Geometry check sheet. Reference: the model listing, model coordinates, mm. A direction names the side the tool comes from. Round coordinates to 2 decimals unless told otherwise and drop trailing zeros. Answer in a Markdown table with one row per item. Add a question column.
from build123d import *

# Parameters (mm, degrees)
SKETCH1_W                                           = 300
SKETCH1_H                                           = 180
BOSS_EXTRUDE1_DEPTH                                 = 10
CBORE_FOR_4_BINDING_HEAD_MACHINE_SCREW1_D           = 3.2639
CBORE_FOR_4_BINDING_HEAD_MACHINE_SCREW1_DEPTH       = 10
CBORE_FOR_4_BINDING_HEAD_MACHINE_SCREW1_CBORE_D     = 6.74624
CBORE_FOR_4_BINDING_HEAD_MACHINE_SCREW1_CBORE_DEPTH = 1.7272


with BuildPart() as part:
    # Sketch1 → Boss-Extrude1 (new body)
    with BuildSketch(Plane(origin=(0, 0, 0), x_dir=(1, 0, 0), z_dir=(0, 1, 0))):
        with Locations((21.639344262, -12.295081967)):
            Rectangle(SKETCH1_W, SKETCH1_H)
    extrude(amount=BOSS_EXTRUDE1_DEPTH)

    # CBORE for #4 Binding Head Machine Screw1
    with Locations(Plane(origin=(0, 10, 0), x_dir=(1, 0, 0), z_dir=(0, 1, 0))):
        with Locations((-123.360655738, 37.704918033), (-123.360655738, -62.295081967), (-78.360655738, -97.295081967), (121.639344262, -97.295081967), (121.639344262, 72.704918033), (166.639344262, 37.704918033), (-78.360655738, 72.704918033)):
            CounterBoreHole(CBORE_FOR_4_BINDING_HEAD_MACHINE_SCREW1_D / 2, CBORE_FOR_4_BINDING_HEAD_MACHINE_SCREW1_CBORE_D / 2, CBORE_FOR_4_BINDING_HEAD_MACHINE_SCREW1_CBORE_DEPTH, depth=CBORE_FOR_4_BINDING_HEAD_MACHINE_SCREW1_DEPTH)


solid = part.part
Item 1: Mould release check, pull along X, two halves, no side actions. Record for faces 1 (the cylindrical face through (163.27, 9.15, -37.85)), 2 (the flat face through (20, 0, 11)), 3 (the flat face through (-128.361, 5, 14)): +X half, -X half, draft (parallel to the pull), parting line (faces both ways), or undercut.
Item 2: Gauge pin test, flat end, axial feed: pin 1 Ø6 at (x, z) = (-78.36, -72.7) entering from +Y. Record the tip position at first contact, or that the pin passes through.
Item 3: Access from +Z, -Z, +X, -X, +Y, -Y to the whole of each face (thin tool, end or side, straight path). Record for faces 4 (the flat face through (20, 5, 102.295)), 5 (the flat face through (123, 8.273, 96)).
Item 4: Scan lines: probe 1 along X at (y, z) = (5, -37.5); probe 2 along Z at (x, y) = (-79.5, 5). Record each from-to range of solid material in increasing order. Write a range as from..to.
Result sheet:
| question | item | result |
|---|---|---|
| 1 | face 1 | undercut |
| 1 | face 2 | draft |
| 1 | face 3 | -X half |
| 2 | pin 1 | stops at y = 8.27 |
| 3 | face 4 | +Z, +X, -X, +Y, -Y |
| 3 | face 5 | +Y |
| 4 | probe 1 | x = -128.36..-124.98, -121.74..165.02, 168.26..171.64 |
| 4 | probe 2 | z = -77.7..-73.87, -71.54..96.13, 98.46..102.3 |
